Can you work these out from the model? Positions are in its coordinate system, mm. Give positions to 0.01 mm unless a question says otherwise; leave off trailing zeros. Order: outer loops, then holes, each group sorted by start corner. A loop starts at its lowest first (then second) coordinate and runs counter-clockwise, first axis right, second up. Notation, with made-up numbers: (49.5, 70.25) - (92.5, 70.25) arc R18 ccw to (92.5, 79.25) - close; hole circle Ø6 at (8.5, 61.5). An arc over 180 degrees is marked (long way). Answer as CSV lines item,"result".
```python
from build123d import *

# Parameters (mm, degrees)
F0_R     = 5
F1_DEPTH = 6
F2_R     = 5
F3_DEPTH = 18.5


with BuildPart() as f1:
    # F0 (on Top) → F1 (new body)
    with BuildSketch(Plane.XY):
        Circle(F0_R)
        with BuildLine():
            ThreePointArc((1.75, 2.185749), (2.523886, 1.212436), (2.8, 0))
            ThreePointArc((2.8, 0), (-1.212436, -2.523886), (-1.75, 2.185749))
            ThreePointArc((-1.75, 2.185749), (0, 2.8), (1.75, 2.185749))
        make_face(mode=Mode.SUBTRACT)
    extrude(amount=F1_DEPTH)

    # F2 (on face) → F3 (join)
    with BuildSketch(Plane.XY.offset(6)):
        Circle(F2_R)
        with BuildLine():
            ThreePointArc((2.8, 0), (-1.268858, -2.495997), (-1.65, 2.262189))
            ThreePointArc((-1.65, 2.262189), (0, 2.8), (1.65, 2.262189))
            ThreePointArc((1.65, 2.262189), (2.495997, 1.268858), (2.8, 0))
        make_face(mode=Mode.SUBTRACT)
        with BuildLine():
            ThreePointArc((1.65, 2.262189), (0, 2.8), (-1.65, 2.262189))
            Line((-1.65, 2.262189), (1.65, 2.262189))
        make_face()
    extrude(amount=F3_DEPTH)


solid = f1.part
```
1) I want a section at A-A on x = 0. Write out the boundary of the cut face in (y, z).
Answer block:
outline,"(-5, 0) - (-2.8, 0) - (-2.8, 24.5) - (-5, 24.5) - close; (2.26, 6) - (2.8, 6) - (2.8, 0) - (5, 0) - (5, 24.5) - (2.26, 24.5) - close"
2) I'm going to push a flat-ended pin straight in: P1, Ø6, axis at x = -3.5, z = 20, coming from the +Y side. Where does the tip first touch, or does it pass through?
Answer block:
P1,"y = 4.97"
3) I need wall thicknesses on line 1 along Y through (x, z) = (0, 15); line 2 along Y through (x, z) = (0, 2); line 3 along X through (y, z) = (1.75, 3.5). Which ranges of each line are inside material? Lowest first, please. Write a range as [from, to].
Answer block:
line 1,"[-5, -2.8], [2.26, 5]"
line 2,"[-5, -2.8], [2.8, 5]"
line 3,"[-4.68, -2.19], [2.19, 4.68]"
4) I want a section at D-D on x = 2.5. Write out the boundary of the cut face in (y, z), plus the area to 3 significant figures.
Answer block:
outline,"(-4.33, 0) - (-1.26, 0) - (-1.26, 24.5) - (-4.33, 24.5) - close; (1.26, 0) - (4.33, 0) - (4.33, 24.5) - (1.26, 24.5) - close"
area,"150 mm2"
5) I want a section at B-B on z = 4. Write out the boundary of the cut face in (x, y), plus the area to 3 significant figures.
Answer block:
outline,"circle Ø10 at (0, 0); hole (-1.75, 2.19) arc R2.8 ccw (long way) to (2.8, 0) arc R2.8 ccw to (1.75, 2.19) arc R2.8 ccw to start"
area,"53.9 mm2"
6) If we mould it in two halves opening along X, with no side actions, what happens to faces 1 (the cylindrical face through (-1.08, -4.88, 12.08)), 2 (the flat face through (0, 2.262, 15)), 3 (the flat face through (2.2, -2.2, 0))? For each: +X half, -X half, draft (parallel to the pull), parting line (faces both ways), or undercut.
Answer block:
face 1,"parting line"
face 2,"undercut"
face 3,"draft"
7) I want a section at C-C on y = -4. Write out the boundary of the cut face in (x, z), plus the area to 3 significant figures.
Answer block:
outline,"(-3, 0) - (3, 0) - (3, 24.5) - (-3, 24.5) - close"
area,"147 mm2"
